Autodesk Inventor part; units mm, degrees
ref_plane "YZ Plane" through (0, 0, 0) normal (1, 0, 0) x (0, 1, 0)
ref_plane "XZ Plane" through (0, 0, 0) normal (0, 1, 0) x (-1, 0, 0)
ref_plane "XY Plane" through (0, 0, 0) normal (0, 0, 1) x (1, 0, 0)
sketch "Esquisse1" plane through (0, 0, 0) normal (0, 0, 1) x (1, 0, 0)
  line L0 (0, 0) -> (170, 0)
  line L1 (170, 0) -> (170, 80)
  line L2 (170, 80) -> (0, 80)
  line L3 (0, 80) -> (0, 0)
  dimension "d0" = 170
  dimension "d1" = 80
extrude "Extrusion1" add sketch "Esquisse1" against normal blind 5
sketch "Esquisse3" plane through (170, 0, 0) normal (1, 0, 0) x (0, 0, -1)
  line L0 (0, 0) -> (0, 80)
  line L1 (0, 80) -> (0, 77.5)
  line L2 (0, 77.5) -> (2.5, 77.5)
  line L3 (0, 77.5) -> (2.5, 77.5) construction
  line L4 (0, 0) -> (2.5, 0)
  line L5 (2.5, 0) -> (2.5, 25)
  dimension "d4" = 2.5
  dimension "d5" = 2.5
  dimension "d6" = 0
  dimension "d14" = 25
hole "Perçage1" at (170, 77.5, -2.5) at (170, 25, -2.5) direction (-1, 0, 0) diameter 2.459 depth 8.8 tip angle 118
sketch "Esquisse4" plane through (0, 0, 0) normal (-1, 0, 0) x (0, 0, 1)
  line L0 (0, 0) -> (-2.5, 0)
  line L1 (0, 0) -> (-5, 0)
  line L2 (-2.5, 0) -> (-2.5, 25)
  line L3 (0, 0) -> (0, 80)
  line L4 (0, 80) -> (-2.5, 80)
  line L5 (-2.5, 80) -> (-2.5, 77.5)
  dimension "d15" = 2.5
  dimension "d16" = 25
  dimension "d17" = 2.5
  dimension "d18" = 90
hole "Perçage2" at (0, 25, -2.5) at (0, 77.5, -2.5) direction (1, 0, 0) diameter 2.459 depth 8.8 tip angle 118
sketch "Esquisse5" plane through (0, 80, 0) normal (0, 1, 0) x (1, 0, 0)
  line L0 (170, 0) -> (0, 0)
  line L1 (170, 5) -> (0, 5)
  point P0 (85, 2.5)
hole "Perçage3" at (85, 80, -2.5) direction (0, -1, 0) diameter 2.459 depth 8.8 tip angle 118
sketch "Esquisse6" plane through (0, 0, 0) normal (0, -1, 0) x (1, 0, 0)
  line L0 (0, 0) -> (170, 0)
  line L1 (0, -5) -> (170, -5)
  point P0 (85, -2.5)
hole "Perçage4" at (85, 0, -2.5) direction (0, 1, 0) diameter 2.459 depth 8.8 tip angle 118
properties part number "chassis_face_arriere"
Could you check a few things on this model? Use its own coordinates, in mm. Give positions to 0.01 mm unless a question says otherwise; leave off trailing zeros.
Item 1: If we mould it in two halves opening along Y, with no side actions, what happens to faces 1 (the face through (86, 80, -4)), 2 (the face through (84, 0, -4)), 3 (the face through (0, 41, -2))? For each: pulls with the +Y half, pulls with the -Y half, needs draft (parallel to the pull), parting line crosses it, or undercut.
Item 2: I'm going to push a flat-ended pin straight in: pin 1 (1.5 mm diameter, centred on y = 77.5, z = -2.5, fed in from -X). Where does the tip first touch, or does it pass through?
Item 3: I need wall thicknesses on line 1 (Y direction, x = 4, z = -2.5); line 2 (Z direction, x = 85, y = 76); line 3 (X direction, y = 26, z = -2). Which ranges of each line are inside material? Lowest first, please.
Values:
1. face 1: pulls with the +Y half
1. face 2: pulls with the -Y half
1. face 3: needs draft
2. pin 1: stops at x = 9.09
3. line 1: y = 0 to 23.77, 26.23 to 76.27, 78.73 to 80
3. line 2: z = -5 to -3.73, -1.27 to 0
3. line 3: x = 8.87 to 161.13
